```python
from build123d import *
from OCP.BRepFilletAPI import BRepFilletAPI_MakeChamfer

# Parameters (mm, degrees)
BOSS_EXTRUDE1_DEPTH = 12.5
SKETCH2_R           = 3.4
CUT_EXTRUDE1_DEPTH  = 122.738705842
SKETCH4_R           = 2.5
BOSS_EXTRUDE2_DEPTH = 8
SKETCH3_R           = 2.9
CUT_EXTRUDE2_DEPTH  = 171.159954161
CUT_EXTRUDE4_REACH  = 127.738
SKETCH8_R           = 2.275
CHAMFER1_SIZE       = 5
CHAMFER1_SIZE2      = 4.195498156
FILLET1_R           = 3
CHAMFER2_SIZE       = 2
CHAMFER2_SIZE2      = 1.400415076
FILLET2_R           = 2


with BuildPart() as part:
    # Sketch1 → Boss-Extrude1 (new, symmetric)
    with BuildSketch(Plane(origin=(0, 0, 0), x_dir=(1, 0, 0), z_dir=(0, 1, 0))):
        Polygon((119.75, 0), (119.75, -7), (47.25, -7), (47.25, -25), (40.25, -25), (40.25, -7), (-40.25, -7), (-40.25, -25), (-47.25, -25), (-47.25, -7), (-72.25, -7), (-72.25, 0), align=None)
    extrude(amount=BOSS_EXTRUDE1_DEPTH, both=True)

    # Sketch2 → Cut-Extrude1 (cut, through all)
    with BuildSketch(Plane.XY.offset(7)):
        with Locations((-60.25, 0)):
            Circle(SKETCH2_R)
        with Locations(Location((60.25, 0, 0), (0, 0, 180))):
            Circle(SKETCH2_R)
    extrude(amount=-CUT_EXTRUDE1_DEPTH, mode=Mode.SUBTRACT)

    # Sketch4 → Boss-Extrude2 (add)
    with BuildSketch(Plane(origin=(0, 12.5, 0), x_dir=(1, 0, 0), z_dir=(0, 1, 0))):
        Polygon((-72.25, -7), (-47.25, -7), (-47.25, -25), (-40.25, -25), (-40.25, -7), (40.25, -7), (40.25, -25), (47.25, -25), (47.25, -7), (72.25, -7), (72.25, 25.4), (-72.25, 25.4), align=None)
        with Locations(Location((-57.25, 12.7, 0), (0, 0, 270))):
            Circle(SKETCH4_R, mode=Mode.SUBTRACT)
        with Locations(Location((57.25, 12.7, 0), (0, 0, 270))):
            Circle(SKETCH4_R, mode=Mode.SUBTRACT)
    extrude(amount=BOSS_EXTRUDE2_DEPTH)

    # Sketch3 → Cut-Extrude2 (cut, through all)
    with BuildSketch(Plane.ZY.offset(47.25)):
        with Locations((17, 4)):
            Circle(SKETCH3_R)
    extrude(amount=-CUT_EXTRUDE2_DEPTH, mode=Mode.SUBTRACT)

    # Sketch8 → Cut-Extrude4 (cut, up to next)
    with BuildSketch(Plane.XY.offset(7), mode=Mode.PRIVATE) as cut_extrude4_sk1:
        with Locations((100.5, 3.5)):
            Circle(SKETCH8_R)
    cut_extrude4_tool1 = extrude(cut_extrude4_sk1.sketch, amount=-CUT_EXTRUDE4_REACH, mode=Mode.PRIVATE) & part.part
    # Sketch8 → Cut-Extrude4 (cut, up to next)
    with BuildSketch(Plane.XY.offset(7), mode=Mode.PRIVATE) as cut_extrude4_sk2:
        with Locations((110.5, 3.5)):
            Circle(SKETCH8_R)
    cut_extrude4_tool2 = extrude(cut_extrude4_sk2.sketch, amount=-CUT_EXTRUDE4_REACH, mode=Mode.PRIVATE) & part.part
    # Sketch8 → Cut-Extrude4 (cut, up to next)
    with BuildSketch(Plane.XY.offset(7), mode=Mode.PRIVATE) as cut_extrude4_sk3:
        with Locations((105.5, -4.5)):
            Circle(SKETCH8_R)
    cut_extrude4_tool3 = extrude(cut_extrude4_sk3.sketch, amount=-CUT_EXTRUDE4_REACH, mode=Mode.PRIVATE) & part.part
    add(cut_extrude4_tool1.solids().sort_by_distance((100.5, 3.5, 7))[0], mode=Mode.SUBTRACT)
    add(cut_extrude4_tool2.solids().sort_by_distance((110.5, 3.5, 7))[0], mode=Mode.SUBTRACT)
    add(cut_extrude4_tool3.solids().sort_by_distance((105.5, -4.5, 7))[0], mode=Mode.SUBTRACT)

    # Chamfer1: one chamfer whose edges measure the first distance from different faces: ONE call of the kernel's chamfer builder (chamfer() names one face for all edges)
    chamfer1_edges_1 = [part.edges().sort_by_distance(p)[0] for p in [
        (119.75, -12.5, 3.5),
        (119.75, 12.5, 3.5),
    ]]
    chamfer1_side_1 = [part.faces().sort_by_distance(p)[0] for p in [
        (119.75, 0, 3.5),
    ]]
    chamfer1_edges_2 = [part.edges().sort_by_distance(p)[0] for p in [
        (43.75, -12.5, 25),
    ]]
    chamfer1_side_2 = [part.faces().sort_by_distance(p)[0] for p in [
        (43.75, 4, 25),
    ]]
    chamfer1_edges_3 = [part.edges().sort_by_distance(p)[0] for p in [
        (-43.75, -12.5, 25),
    ]]
    chamfer1_side_3 = [part.faces().sort_by_distance(p)[0] for p in [
        (-43.75, 4, 25),
    ]]
    chamfer1_edges_4 = [part.edges().sort_by_distance(p)[0] for p in [
        (-72.25, -12.5, 3.5),
    ]]
    chamfer1_side_4 = [part.faces().sort_by_distance(p)[0] for p in [
        (-72.25, 4, 6.537532704),
    ]]
    chamfer1 = BRepFilletAPI_MakeChamfer(part.part.solid().wrapped)
    for e in chamfer1_edges_1:
        chamfer1.Add(CHAMFER1_SIZE, CHAMFER1_SIZE2, e.wrapped, chamfer1_side_1[0].wrapped)  # the first distance lies on this face
    for e in chamfer1_edges_2:
        chamfer1.Add(CHAMFER1_SIZE, CHAMFER1_SIZE2, e.wrapped, chamfer1_side_2[0].wrapped)  # the first distance lies on this face
    for e in chamfer1_edges_3:
        chamfer1.Add(CHAMFER1_SIZE, CHAMFER1_SIZE2, e.wrapped, chamfer1_side_3[0].wrapped)  # the first distance lies on this face
    for e in chamfer1_edges_4:
        chamfer1.Add(CHAMFER1_SIZE, CHAMFER1_SIZE2, e.wrapped, chamfer1_side_4[0].wrapped)  # the first distance lies on this face
    add(Compound.cast(chamfer1.Shape()), mode=Mode.REPLACE)

    # Fillet1
    fillet1_edges = [part.edges().sort_by_distance(p)[0] for p in [
        (115.554501844, 12.5, 3.5),
        (119.75, -7.5, 3.5),
        (-43.75, -12.5, 20.804501844),
        (43.75, -12.5, 20.804501844),
        (-68.054501844, -12.5, 3.5),
        (115.554501844, -12.5, 3.5),
        (-72.25, -7.5, 3.5),
        (43.75, -7.5, 25),
        (-43.75, -7.5, 25),
    ]]
    fillet(fillet1_edges, radius=FILLET1_R)

    # Chamfer2: one chamfer whose edges measure the first distance from different faces: ONE call of the kernel's chamfer builder (chamfer() names one face for all edges)
    chamfer2_edges_1 = [part.edges().sort_by_distance(p)[0] for p in [
        (-72.25, 20.5, -9.2),
    ]]
    chamfer2_side_1 = [part.faces().sort_by_distance(p)[0] for p in [
        (-72.25, 7.045955351, 6.578834324),
    ]]
    chamfer2_edges_2 = [part.edges().sort_by_distance(p)[0] for p in [
        (-59.75, 20.5, 7),
    ]]
    chamfer2_side_2 = [part.faces().sort_by_distance(p)[0] for p in [
        (-59.571971044, 4.394421722, 7),
    ]]
    chamfer2_edges_3 = [part.edges().sort_by_distance(p)[0] for p in [
        (-47.25, 20.5, 16),
    ]]
    chamfer2_side_3 = [part.faces().sort_by_distance(p)[0] for p in [
        (-47.25, -12.124101077, 13.202789435),
    ]]
    chamfer2_edges_4 = [part.edges().sort_by_distance(p)[0] for p in [
        (-40.25, 20.5, 16),
    ]]
    chamfer2_side_4 = [part.faces().sort_by_distance(p)[0] for p in [
        (-40.25, -12.124101077, 13.202789435),
    ]]
    chamfer2_edges_5 = [part.edges().sort_by_distance(p)[0] for p in [
        (0, 20.5, 7),
    ]]
    chamfer2_side_5 = [part.faces().sort_by_distance(p)[0] for p in [
        (0, 4, 7),
    ]]
    chamfer2_edges_6 = [part.edges().sort_by_distance(p)[0] for p in [
        (40.25, 20.5, 16),
    ]]
    chamfer2_side_6 = [part.faces().sort_by_distance(p)[0] for p in [
        (40.25, -12.124101077, 13.202789435),
    ]]
    chamfer2_edges_7 = [part.edges().sort_by_distance(p)[0] for p in [
        (47.25, 20.5, 16),
    ]]
    chamfer2_side_7 = [part.faces().sort_by_distance(p)[0] for p in [
        (47.25, -12.124101077, 13.202789435),
    ]]
    chamfer2_edges_8 = [part.edges().sort_by_distance(p)[0] for p in [
        (59.75, 20.5, 7),
    ]]
    chamfer2_side_8 = [part.faces().sort_by_distance(p)[0] for p in [
        (80.49228868, 1.71079357, 7),
    ]]
    chamfer2 = BRepFilletAPI_MakeChamfer(part.part.solid().wrapped)
    for e in chamfer2_edges_1:
        chamfer2.Add(CHAMFER2_SIZE, CHAMFER2_SIZE2, e.wrapped, chamfer2_side_1[0].wrapped)  # the first distance lies on this face
    for e in chamfer2_edges_2:
        chamfer2.Add(CHAMFER2_SIZE, CHAMFER2_SIZE2, e.wrapped, chamfer2_side_2[0].wrapped)  # the first distance lies on this face
    for e in chamfer2_edges_3:
        chamfer2.Add(CHAMFER2_SIZE, CHAMFER2_SIZE2, e.wrapped, chamfer2_side_3[0].wrapped)  # the first distance lies on this face
    for e in chamfer2_edges_4:
        chamfer2.Add(CHAMFER2_SIZE, CHAMFER2_SIZE2, e.wrapped, chamfer2_side_4[0].wrapped)  # the first distance lies on this face
    for e in chamfer2_edges_5:
        chamfer2.Add(CHAMFER2_SIZE, CHAMFER2_SIZE2, e.wrapped, chamfer2_side_5[0].wrapped)  # the first distance lies on this face
    for e in chamfer2_edges_6:
        chamfer2.Add(CHAMFER2_SIZE, CHAMFER2_SIZE2, e.wrapped, chamfer2_side_6[0].wrapped)  # the first distance lies on this face
    for e in chamfer2_edges_7:
        chamfer2.Add(CHAMFER2_SIZE, CHAMFER2_SIZE2, e.wrapped, chamfer2_side_7[0].wrapped)  # the first distance lies on this face
    for e in chamfer2_edges_8:
        chamfer2.Add(CHAMFER2_SIZE, CHAMFER2_SIZE2, e.wrapped, chamfer2_side_8[0].wrapped)  # the first distance lies on this face
    add(Compound.cast(chamfer2.Shape()), mode=Mode.REPLACE)

    # Fillet2
    fillet2_edges = [part.edges().sort_by_distance(p)[0] for p in [
        (-72.25, 6.045955351, 7),
        (-72.069077862, -7.434149727, 7),
        (-70.250922764, -9.882407478, 7),
        (-67.923433655, -12.218923361, 7),
        (-56.952789435, -12.5, 7),
        (119.569077862, -7.434149727, 7),
        (117.750922764, -9.882407478, 7),
        (115.423433655, -12.218923361, 7),
        (119.75, 0.545955351, 0),
        (119.569077862, -7.434149727, 0),
        (117.750922764, -9.882407478, 0),
        (115.423433655, -12.218923361, 0),
        (-72.25, 3.045955351, 0),
        (-72.069077862, -7.434149727, 0),
        (-70.250922764, -9.882407478, 0),
        (-67.923433655, -12.218923361, 0),
        (47.25, -12.5, 13.202789435),
        (47.25, -12.218923361, 20.673433655),
        (47.25, -9.882407478, 23.000922764),
        (47.25, -7.434149727, 24.819077862),
        (40.25, -12.5, 13.202789435),
        (40.25, -12.218923361, 20.673433655),
        (40.25, -9.882407478, 23.000922764),
        (40.25, -7.434149727, 24.819077862),
        (-40.25, -12.5, 13.202789435),
        (-40.25, -12.218923361, 20.673433655),
        (-40.25, -9.882407478, 23.000922764),
        (-40.25, -7.434149727, 24.819077862),
        (-47.25, -12.5, 13.202789435),
        (-47.25, -12.218923361, 20.673433655),
        (-47.25, -9.882407478, 23.000922764),
        (-47.25, -7.434149727, 24.819077862),
        (-47.25, 6.045955351, 25),
        (47.25, 3, 7),
        (80.702789435, -12.5, 7),
        (0, -12.5, 7),
        (23.75, -12.5, 0),
        (-47.25, 3, 7),
        (47.25, 6.045955351, 25),
        (40.25, 6.045955351, 25),
        (-40.25, 6.045955351, 25),
        (119.75, 0.545955351, 7),
    ]]
    fillet(fillet2_edges, radius=FILLET2_R)


solid = part.part
```
Verification items for the finished model (mm, model axes). A direction names the side the tool comes from. Give positions to 0.01 mm unless a question says otherwise; leave off trailing zeros. Order: outer loops, then holes, each group sorted by start corner. A loop starts at its lowest first (then second) coordinate and runs counter-clockwise, first axis right, second up. Notation, with made-up numbers: M -33,7 L 14,7 A9 cw 14,23 Z; hole C -9.75,0 d2. An arc over 180 degrees is marked long. Answer in a Markdown table with one row per item. Add a question column.
Item 1: Section check B-B, the plane z = 17. Enter the section's corners in (x, y), and give its area (3 significant figures).
Item 2: Mould release check, pull along Y, two halves, no side actions. Record for faces 1 (the flat face through (17, -12.5, 4)), 2 (the flat face through (1, 16, -25.4)), 3 (the cylindrical face through (-57, -1, 4)): released by +Y, released by -Y, zero draft, split by the parting line, or undercut.
Item 3: Section check C-C, the plane x = 51. Enter the section's corners in (y, z).
Item 4: Section check D-D, the plane z = -3. Enter the section's corners in (x, y), and give its area (3 significant figures).
Item 5: Section check A-A, the plane x = 105.5. Enter the section's corners in (y, z) (3 decimals), and give its area (3 significant figures).
Item 6: Tool access check on faces 4 (the flat face through (-40.25, 4, 13)), 5 (the flat face through (93, 12.5, 3)), 6 (the cylindrical face through (40.851, -9.537, 22.546)), 7 (the flat face through (-47.25, 4, 13)), 8 (the flat face through (47.25, 4, 13)). Record the directions out of +Z, -Z, +X, -X, +Y, -Y that give a thin tool (end or side, any length) a straight path to the whole face; none if there is none.
Item 7: Gauge pin test, flat ends, axial feed: pin 1 (6.5 mm diameter, centred on x = -63, y = 4, fed in from +Z); pin 2 (6.5 mm diameter, centred on y = 4, z = 17, fed in from +X); pin 3 (13.5 mm diameter, centred on x = -22.5, z = -9.5, fed in from -Y). Record the tip position at first contact, or that the pin passes through.
Item 8: Scan lines: probe 1 along X at (y, z) = (17.5, -12.7); probe 2 along X at (y, z) = (10, 22); probe 3 along Y at (x, z) = (43, 17). Record each from-to range of solid material in increasing order. Write a range as from..to.
Filled sheet:
| question | item | result |
|---|---|---|
| 1 | outline | M -47.25,-10.5 A2 ccw -45.25,-12.5 L -42.25,-12.5 A2 ccw -40.25,-10.5 L -40.25,1.1 L -47.25,1.1 Z; M -47.25,6.9 L -40.25,6.9 L -40.25,18.5 L -41.65,20.5 L -45.85,20.5 L -47.25,18.5 Z; M 40.25,-10.5 A2 ccw 42.25,-12.5 L 45.25,-12.5 A2 ccw 47.25,-10.5 L 47.25,1.1 L 40.25,1.1 Z; M 40.25,6.9 L 47.25,6.9 L 47.25,18.5 L 45.85,20.5 L 41.65,20.5 L 40.25,18.5 Z |
| 1 | area | 372 mm^2 |
| 2 | face 1 | released by -Y |
| 2 | face 2 | zero draft |
| 2 | face 3 | undercut |
| 3 | outline | M -12.5,2 A2 ccw -10.5,0 L 12.5,0 L 12.5,-25.4 L 20.5,-25.4 L 20.5,5.6 L 18.5,7 L -10.5,7 A2 ccw -12.5,5 Z |
| 4 | outline | M -72.25,12.5 L 72.25,12.5 L 72.25,20.5 L -70.85,20.5 L -72.25,18.5 Z |
| 4 | area | 1,150 mm^2 |
| 5 | outline | M -12.5,2 A2 ccw -10.5,0 L -6.775,0 L -6.775,7 L -10.5,7 A2 ccw -12.5,5 Z; M -2.225,0 L 12.5,0 L 12.5,7 L -2.225,7 Z |
| 5 | area | 141 mm^2 |
| 6 | face 4 | +Z, +Y, -Y |
| 6 | face 5 | +Z, -Z, +X, +Y |
| 6 | face 6 | +Z, -Y |
| 6 | face 7 | +Z, -X, +Y, -Y |
| 6 | face 8 | +Z, +X, +Y, -Y |
| 7 | pin 1 | stops at z = 7 |
| 7 | pin 2 | stops at x = 47.25 |
| 7 | pin 3 | stops at y = 12.5 |
| 8 | probe 1 | x = -72.25..-59.75, -54.75..54.75, 59.75..72.25 |
| 8 | probe 2 | x = -47.25..-40.25, 40.25..47.25 |
| 8 | probe 3 | y = -12.5..1.1, 6.9..20.5 |
